For this review, take the finished solid that the model builds, in its own axes (mm). A direction names the side the tool comes from. Coordinates: 2 decimals unless noted, no trailing zeros. Loops run counter-clockwise (first coordinate to the right, second up) from the corner with the lowest first, then second, coordinate; pieces in that order, holes last.
1. Mouldability with a two-part tool opening along X and no side actions: class faces 1 (the face through (-2.685, 2.274, -0.596)), 2 (the face through (-2, 4.5, 3)), 3 (the face through (-9.76, 0.99, -2.17)) as pulls with the +X half, pulls with the -X half, needs draft (parallel to the pull), parting line crosses it, or undercut.
2. Clearance check with flat-ended pins moving along their axes: P1, Ø1.6, axis at x = 1, z = 0, coming from the +Y side; P2, Ø2, axis at y = 2.5, z = -7.5, coming from the -X side; P3, Ø1, axis at y = 1.5, z = -6.5, coming from the -X side. State where each tip first meets the part, or that it passes through.
3. Take a section at C-C, the plane y = 1.5. State the section outline as (x, z) points, then the cut area to 3 significant figures.
4. To check wall thickness, follow probe 1 along X at (y, z) = (0.6, 0); probe 2 along X at (y, z) = (0.4, 0); probe 3 along X at (y, z) = (2.3, 0). State the ranges of each line that lie inside material, in increasing order.
5. Take a section at A-A, the plane z = 0. State the section outline as (x, y) points, then the cut area to 4 significant figures.
6. Take a section at B-B, the plane x = 8. State the section outline as (y, z) points, then the cut area to 3 significant figures.
7. Take a section at D-D, the plane z = -6.5. State the section outline as (x, y) points.
8. Machinability: for faces 4 (the face through (-1.2, 0.5, 1.2)), 5 (the face through (-2, 0, 0)), which of the approach directions +Z, -Z, +X, -X, +Y, -Y give a long, thin tool a straight path to every point of the face, cutting with its end or side? Answer none if there is none.
```python
from build123d import *

# Parameters (mm, degrees)
SKETCH_1_R          = 10
EXTRUDE_1_DEPTH     = 2
SKETCH_2_R          = 1.5
CUT_EXTRUDE_1_DEPTH = 2
SKETCH_3_R          = 4.5
EXTRUDE_2_DEPTH     = 2.5
SKETCH_4_R          = 2.75
CUT_EXTRUDE_2_DEPTH = 4
SKETCH_5_R          = 1.5
CUT_EXTRUDE_3_DEPTH = 4
CHAMFER_1_SIZE      = 0.5


with BuildPart() as part:
    # 草图1 → 凸台-拉伸1 (new body)
    with BuildSketch(Plane(origin=(0, 0, 0), x_dir=(1, 0, 0), z_dir=(0, 1, 0))):
        with Locations(Location((0, 0, 0), (0, 0, 270))):
            Circle(SKETCH_1_R)
    extrude(amount=EXTRUDE_1_DEPTH)

    # 草图2 → 切除-拉伸1 (cut)
    with BuildSketch(Plane(origin=(0, 2, 0), x_dir=(1, 0, 0), z_dir=(0, 1, 0))):
        with Locations(Location((-7, 0, 0), (0, 0, 270))):
            Circle(SKETCH_2_R)
        with Locations(Location((0, 7, 0), (0, 0, 270))):
            Circle(SKETCH_2_R)
        with Locations(Location((7, 0, 0), (0, 0, 270))):
            Circle(SKETCH_2_R)
        with Locations(Location((0, -7, 0), (0, 0, 270))):
            Circle(SKETCH_2_R)
    extrude(amount=-CUT_EXTRUDE_1_DEPTH, mode=Mode.SUBTRACT)

    # 草图3 → 凸台-拉伸2 (add)
    with BuildSketch(Plane(origin=(0, 2, 0), x_dir=(1, 0, 0), z_dir=(0, 1, 0))):
        with Locations(Location((0, 0, 0), (0, 0, 270))):
            Circle(SKETCH_3_R)
    extrude(amount=EXTRUDE_2_DEPTH)

    # 草图4 → 切除-拉伸2 (cut)
    with BuildSketch(Plane(origin=(0, 4.5, 0), x_dir=(1, 0, 0), z_dir=(0, 1, 0))):
        with Locations(Location((0, 0, 0), (0, 0, 270))):
            Circle(SKETCH_4_R)
    extrude(amount=-CUT_EXTRUDE_2_DEPTH, mode=Mode.SUBTRACT)

    # 草图5 → 切除-拉伸3 (cut)
    with BuildSketch(Plane(origin=(0, 0.5, 0), x_dir=(1, 0, 0), z_dir=(0, 1, 0))):
        with Locations(Location((0, 0, 0), (0, 0, 270))):
            Circle(SKETCH_5_R)
    extrude(amount=-CUT_EXTRUDE_3_DEPTH, mode=Mode.SUBTRACT)

    # 倒角1
    chamfer_1_edges = [part.edges().sort_by_distance(p)[0] for p in [
        (0, 4.5, -2.75),
    ]]
    chamfer(chamfer_1_edges, length=CHAMFER_1_SIZE)


solid = part.part
```
Results list:
1. face 1: undercut
1. face 2: needs draft
1. face 3: parting line crosses it
2. P1: stops at y = 0.5
2. P2: stops at x = -7.48
2. P3: stops at x = -8
3. outline: circle Ø20 at (0, 0); hole circle Ø3 at (-7, 0); hole circle Ø5.5 at (0, 0); hole circle Ø3 at (0, -7); hole circle Ø3 at (0, 7); hole circle Ø3 at (7, 0)
3. area: 262 mm2
4. probe 1: x = -10 to -8.5, -5.5 to -2.75, 2.75 to 5.5, 8.5 to 10
4. probe 2: x = -10 to -8.5, -5.5 to -1.5, 1.5 to 5.5, 8.5 to 10
4. probe 3: x = -4.5 to -2.75, 2.75 to 4.5
5. outline: (-10, 0) - (-8.5, 0) - (-8.5, 2) - (-10, 2) - close; (-5.5, 0) - (-1.5, 0) - (-1.5, 0.5) - (-2.75, 0.5) - (-2.75, 4) - (-3.25, 4.5) - (-4.5, 4.5) - (-4.5, 2) - (-5.5, 2) - close; (1.5, 0) - (5.5, 0) - (5.5, 2) - (4.5, 2) - (4.5, 4.5) - (3.25, 4.5) - (2.75, 4) - (2.75, 0.5) - (1.5, 0.5) - close; (8.5, 0) - (10, 0) - (10, 2) - (8.5, 2) - close
5. area: 26.75 mm2
6. outline: (0, -6) - (2, -6) - (2, -1.12) - (0, -1.12) - close; (0, 1.12) - (2, 1.12) - (2, 6) - (0, 6) - close
6. area: 19.5 mm2
7. outline: (-7.6, 0) - (-1.41, 0) - (-1.41, 2) - (-7.6, 2) - close; (1.41, 0) - (7.6, 0) - (7.6, 2) - (1.41, 2) - close
8. face 4: +Y
8. face 5: +Z, -Z, +X, -X, -Y
